Drawing for the job (mm, zero at the part's lowest x, y, z). Give positions to 0.01 mm unless a question says otherwise; leave off trailing zeros. Order: outer loops, then holes, each group sorted by start corner. A loop starts at its lowest first (then second) coordinate and runs counter-clockwise, first axis right, second up. Notation, with made-up numbers: (60, 42.25) - (104, 42.25) arc R17 ccw to (104, 67.25) - close; hole circle Ø9 at (68, 35). An arc over 180 degrees is marked (long way). Use a Markdown table: item, result. Add a question column.
(1) Slice it at A-A (y = 184.15). Write the cut outline in (x, z) (1 decimal).
(2) Slice it at C-C (y = 162). Write the cut outline in (x, z) (1 decimal), then the cut area to 3 significant figures.
(3) Flat gauge pins, fed straight in: pin 1 (0.8 mm diameter, centred on x = 9, z = 3, fed in from +Y); pin 2 (6 mm diameter, centred on y = 152, z = 12.5, fed in from +X); pin 3 (2 mm diameter, centred on y = 159, z = 14, fed in from -X); pin 4 (2.5 mm diameter, centred on y = 184.15, z = 7.94, fed in from -X). Where does each tip first touch, or does it go through?
(4) Slice it at B-B (z = 13.75). Count the separate pieces of the cut face and the enclosed holes in it, then the cut area to 3 significant figures.
(5) Wall check: line 1 (Y direction, x = 2.75, z = 11.25) (1 decimal); line 2 (Y direction, x = 5, z = 8) (1 decimal); line 3 (X direction, y = 171.45, z = 10) (1 decimal). Give the ranges that are in metal, low to high.
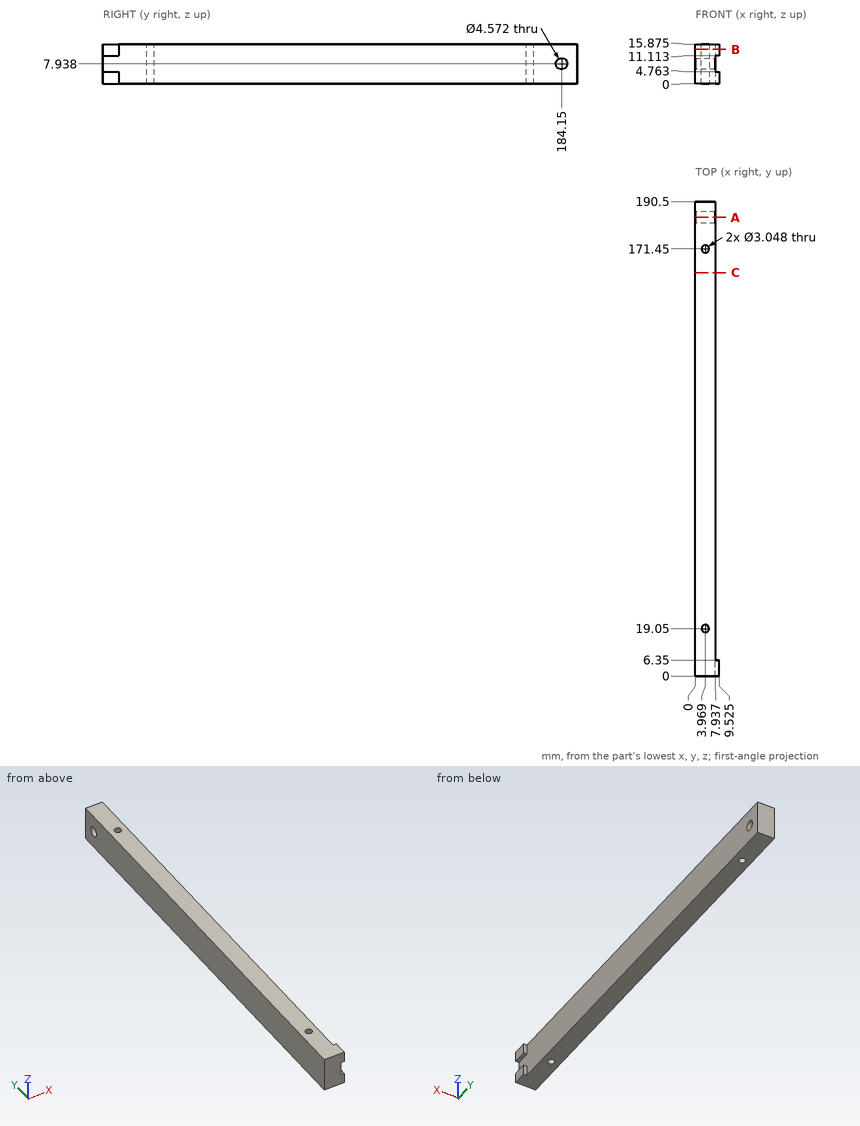
Solution:
| question | item | result |
|---|---|---|
| 1 | outline | (0, 0) - (7.9, 0) - (7.9, 5.7) - (0, 5.7) - close; (0, 10.2) - (7.9, 10.2) - (7.9, 15.9) - (0, 15.9) - close |
| 2 | outline | (0, 0) - (7.9, 0) - (7.9, 15.9) - (0, 15.9) - close |
| 2 | area | 126 mm2 |
| 3 | pin 1 | y = 6.35 |
| 3 | pin 2 | x = 7.94 |
| 3 | pin 3 | x = 0 |
| 3 | pin 4 | through |
| 4 | separate pieces | 1 |
| 4 | enclosed holes | 2 |
| 4 | area | 1,510 mm2 |
| 5 | line 1 | 0 to 18.1, 20 to 170.5, 172.4 to 190.5 |
| 5 | line 2 | 0 to 17.9, 20.2 to 170.3, 172.6 to 181.9, 186.4 to 190.5 |
| 5 | line 3 | 0 to 2.4, 5.5 to 7.9 |
